Read the model definition and answer for the solid it produces. Units are mm, in the model's axes. Give positions to 0.01 mm unless a question says otherwise; leave off trailing zeros. Loops run counter-clockwise (first coordinate to the right, second up) from the corner with the lowest first, then second, coordinate; pieces in that order, holes last. Notation, with made-up numbers: (-37, -18) - (-31, -18) arc R17 ccw to (-31, -11) - close; hole circle Ø6 at (60, 32.25). An arc over 180 degrees is marked (long way). Use a Markdown table: item, result. Add a question column.
Item 1: Consider probe 1 along Y at (x, z) = (0, 0.3); probe 2 along Y at (x, z) = (-6.5, 0.7); probe 3 along Y at (x, z) = (-13.5, 0.6). Determine where each line is inside the solid, lowest interval first. Write a range as [from, to].
Item 2: This flat-tipped pin is pushed along its axis until it touches: P1, Ø5, axis at x = 41.01, y = 41.01, coming from the -Z side. Where does it stop, or does it pass through?
Item 3: A cutting plane is placed at B-B (x = -34.5). Determine the outline of the cut face in (y, z).
Item 4: A cutting plane is placed at D-D (z = 0.65). Give the number of separate pieces and of enclosed holes in the cut face, plus the area to 3 significant figures.
Item 5: A cutting plane is placed at A-A (y = -23). Determine the outline of the cut face in (x, z).
Item 6: A cutting plane is placed at C-C (y = 0). Determine the outline of the cut face in (x, z), plus the area to 3 significant figures.
from build123d import *

# Parameters (mm, degrees)
SKETCH_R      = 65
SKETCH_R_2    = 50
SKETCH_R_3    = 1.5
EXTRUDE_DEPTH = 1


with BuildPart() as part:
    # Sketch → Extrude (new body)
    with BuildSketch(Plane.XY):
        Circle(SKETCH_R)
        Circle(SKETCH_R_2, mode=Mode.SUBTRACT)
        with Locations((-41.012193, 41.012193)):
            Circle(SKETCH_R_3, mode=Mode.SUBTRACT)
        with Locations((0, 58)):
            Circle(SKETCH_R_3, mode=Mode.SUBTRACT)
        with Locations((58, 0)):
            Circle(SKETCH_R_3, mode=Mode.SUBTRACT)
        with Locations((0, -58)):
            Circle(SKETCH_R_3, mode=Mode.SUBTRACT)
        with Locations((-41.012193, -41.012193)):
            Circle(SKETCH_R_3, mode=Mode.SUBTRACT)
        with Locations((-58, 0)):
            Circle(SKETCH_R_3, mode=Mode.SUBTRACT)
        with Locations((41.012193, -41.012193)):
            Circle(SKETCH_R_3, mode=Mode.SUBTRACT)
        with Locations((41.012193, 41.012193)):
            Circle(SKETCH_R_3, mode=Mode.SUBTRACT)
    extrude(amount=EXTRUDE_DEPTH)


solid = part.part
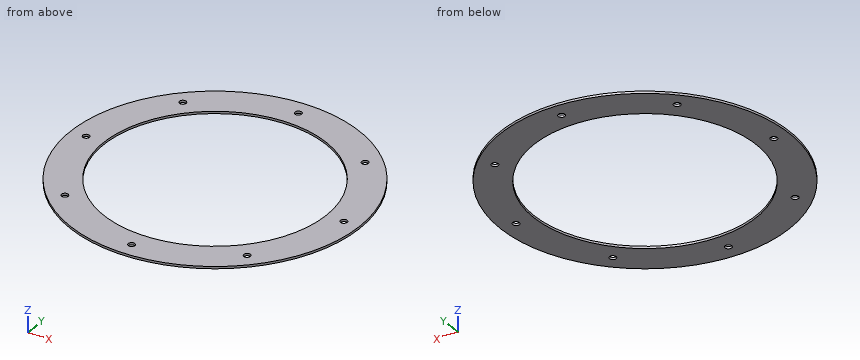
Geometry says:
| question | item | result |
|---|---|---|
| 1 | probe 1 | [-65, -59.5], [-56.5, -50], [50, 56.5], [59.5, 65] |
| 1 | probe 2 | [-64.67, -49.58], [49.58, 64.67] |
| 1 | probe 3 | [-63.58, -48.14], [48.14, 63.58] |
| 2 | P1 | z = 0 |
| 3 | outline | (-55.09, 0) - (-36.19, 0) - (-36.19, 1) - (-55.09, 1) - close; (36.19, 0) - (55.09, 0) - (55.09, 1) - (36.19, 1) - close |
| 4 | separate pieces | 1 |
| 4 | enclosed holes | 9 |
| 4 | area | 5,360 mm² |
| 5 | outline | (-60.79, 0) - (-44.4, 0) - (-44.4, 1) - (-60.79, 1) - close; (44.4, 0) - (60.79, 0) - (60.79, 1) - (44.4, 1) - close |
| 6 | outline | (-65, 0) - (-59.5, 0) - (-59.5, 1) - (-65, 1) - close; (-56.5, 0) - (-50, 0) - (-50, 1) - (-56.5, 1) - close; (50, 0) - (56.5, 0) - (56.5, 1) - (50, 1) - close; (59.5, 0) - (65, 0) - (65, 1) - (59.5, 1) - close |
| 6 | area | 24.0 mm² |
